Autodesk Inventor part; units mm, degrees
ref_plane "YZ Plane" through (0, 0, 0) normal (1, 0, 0) x (0, 1, 0)
ref_plane "XZ Plane" through (0, 0, 0) normal (0, 1, 0) x (-1, 0, 0)
ref_plane "XY Plane" through (0, 0, 0) normal (0, 0, 1) x (1, 0, 0)
sketch "Sketch4" plane through (0, 0, 0) normal (0, 1, 0) x (-1, 0, 0)
  line L0 (17, 17) -> (-17, 17)
  line L1 (-17, 17) -> (-17, -17)
  line L2 (-17, -17) -> (17, -17)
  line L3 (17, -17) -> (17, 17)
  line L4 (17, 17) -> (-17, -17) construction
  line L5 (-17, 17) -> (17, -17) construction
  point P0 (0, 0)
  dimension "d52" = 34
  dimension "d53" = 34
extrude "Extrusion5" add sketch "Sketch4" along normal blind 2
sketch "Sketch6" plane through (0, 0, 0) normal (0, -1, 0) x (1, 0, 0)
  line L0 (-16.5, -10) -> (-15.5, -10)
  line L1 (-15.5, -10) -> (-15.5, 10)
  line L2 (-15.5, 10) -> (-16.5, 10)
  line L3 (-16.5, 10) -> (-16.5, -10)
  line L4 (-15.5, -10) -> (-16.5, -10)
  line L5 (-16.5, -10) -> (-16.5, 10)
  line L6 (-16.5, 10) -> (-15.5, 10)
  line L7 (-15.5, 10) -> (-15.5, -10)
  line L8 (-10, 16.5) -> (10, 16.5)
  line L9 (10, 16.5) -> (10, 15.5)
  line L10 (10, 15.5) -> (-10, 15.5)
  line L11 (-10, 15.5) -> (-10, 16.5)
  line L12 (10, 16.5) -> (-10, 16.5)
  line L13 (-10, 16.5) -> (-10, 15.5)
  line L14 (-10, 15.5) -> (10, 15.5)
  line L15 (10, 15.5) -> (10, 16.5)
  line L16 (15.5, 10) -> (16.5, 10)
  line L17 (16.5, 10) -> (16.5, -10)
  line L18 (16.5, -10) -> (15.5, -10)
  line L19 (15.5, -10) -> (15.5, 10)
  line L20 (15.5, -10) -> (16.5, -10)
  line L21 (16.5, -10) -> (16.5, 10)
  line L22 (16.5, 10) -> (15.5, 10)
  line L23 (15.5, 10) -> (15.5, -10)
  line L24 (10, -15.5) -> (-10, -15.5)
  line L25 (-10, -15.5) -> (-10, -16.5)
  line L26 (-10, -16.5) -> (10, -16.5)
  line L27 (10, -16.5) -> (10, -15.5)
  line L28 (-10, -15.5) -> (10, -15.5)
  line L29 (10, -15.5) -> (10, -16.5)
  line L30 (10, -16.5) -> (-10, -16.5)
  line L31 (-10, -16.5) -> (-10, -15.5)
  line L32 (-17, 17) -> (-17, -17)
  line L33 (17, 17) -> (-17, 17)
  line L34 (17, -17) -> (17, 17)
  line L35 (-17, -17) -> (17, -17)
  line L36 (17, 17) -> (17, -17)
  line L37 (-17, -17) -> (-17, 17)
  line L38 (-17, 17) -> (17, 17)
  line L39 (17, -17) -> (-17, -17)
  point P0 (0, 0)
  point P1 (-16, 10)
  point P2 (-16, -10)
  point P3 (16, 10)
  point P4 (16, -10)
  point P5 (-10, -16)
  point P6 (-16, -10)
  dimension "d123" = 1
  dimension "d124" = 20
  dimension "d119" = 1
  dimension "d118" = 20
  dimension "d116" = 20
  dimension "d117" = 1
  dimension "d112" = 20
  dimension "d113" = 1
  dimension "d108" = 1
  dimension "d109" = 20
  dimension "d104" = 1
  dimension "d105" = 20
  dimension "d101" = 20
  dimension "d102" = 1
  dimension "d97" = 20
  dimension "d98" = 1
  dimension "d114" = 7
  dimension "d115" = 0.5
  dimension "d111" = 0.5
  dimension "d110" = 7
  dimension "d107" = 7
  dimension "d106" = 0.5
  dimension "d103" = 0.5
  dimension "d95" = 7
  dimension "d99" = 7
  dimension "d100" = 0.5
  dimension "d96" = 0.5
  dimension "d94" = 7
  dimension "d93" = 7
  dimension "d122" = 0.5
  dimension "d120" = 7
  dimension "d121" = 0.5
  dimension "d133" = 0
  dimension "d134" = 0
  dimension "d135" = 0
  dimension "d136" = 0
extrude "Extrusion7" add sketch "Sketch6" along normal blind 1 contours L3 L2 L1 L0 | L8 L9 L10 L11 | L16 L17 L18 L19 | L27 L26 L25 L24
fillet "Fillet9" radius 1 1 edges at (17, 1, -17)
fillet "Fillet10" radius 1 1 edges at (-17, 1, -17)
fillet "Fillet11" radius 1 1 edges at (-17, 1, 17)
fillet "Fillet12" radius 1 1 edges at (17, 1, 17)
fillet "Fillet13" radius 1 8 edges at (-16.7071, 2, -16.7071) (-17, 2, 0) (-16.7071, 2, 16.7071) (0, 2, 17) (16.7071, 2, 16.7071) (17, 2, 0) (16.7071, 2, -16.7071) (0, 2, -17)
properties part number "block_main" material "PC/ABS Plastic"
Can you work these out from the model? Positions are in its coordinate system, mm. A direction names the side the tool comes from. Give positions to 0.01 mm unless a question says otherwise; leave off trailing zeros. Write each loop counter-clockwise with the first axis right and the second up, starting at its lowest first coordinate (ties: lowest second). Pieces come first, ordered by that corner, then holes. Notation, with made-up numbers: (23, -18) -> (43, -18) arc R30 ccw to (43, 7) -> close; hole circle Ø8 at (-9.5, 36.25). An arc over 180 degrees is marked (long way). Answer as a JSON object with one key per item and string values. Group by question number.
Item 1: We'd pull the mould along X, two halves only. Please class faces 6 (the face through (-15.5, -0.5, -0.1)), 7 (the face through (0.1, -0.5, 15.5)), 8 (the face through (16.5, -0.5, 0.1)): +X half, -X half, draft (parallel to the pull), parting line (faces both ways), or undercut.
Item 2: For faces 1 (the face through (-16, -0.5, 10)), 2 (the face through (16.699, 1.715, -0.224)), 3 (the face through (0.1, -0.5, -15.5)), 4 (the face through (-16, -0.5, -10)), 5 (the face through (16, -1, 0)), which set-ups out of +Z, -Z, +X, -X, +Y, -Y let a thin tool reach every point of the face, with its end or its side?
Item 3: Suppose I cut it at C-C (y = 1.6). Please give me the cut outline in (x, z).
Item 4: I'm going to push flat-ended pins straight in: P1, Ø0.5, axis at y = -0.5, z = 16, coming from the +X side; P2, Ø3, axis at x = -8, z = -9.5, coming from the -Y side; P3, Ø0.8, axis at x = -16, y = -0.5, coming from the +Z side. Where does each tip first touch, or does it pass through?
Item 5: Please list where these lines run through material, in increasing order: line 1 (Z direction, x = 9, y = -0.15); line 2 (Y direction, x = 2, z = -11). Write a range as [from, to].
Item 6: Suppose I cut it at D-D (x = 4). Please give me the cut outline in (y, z), plus the area to 3 significant figures.
Item 7: Suppose I cut it at A-A (y = -0.4). Please give me the cut outline in (x, z), plus the area to 3 significant figures.
Item 8: Suppose I cut it at B-B (z = 8). Please give me the cut outline in (x, y), plus the area to 3 significant figures.
Findings:
{
 "1": {"face 6": "undercut", "face 7": "draft", "face 8": "+X half"},
 "2": {"face 1": "+Z, +X, -X, -Y", "face 2": "+Z, -Z, +X, +Y", "face 3": "+X, -X, -Y", "face 4": "-Z, +X, -X, -Y", "face 5": "+Z, -Z, +X, -X, -Y"},
 "3": {"outline": "(-16.8, -16) arc R0.8 ccw to (-16, -16.8) -> (16, -16.8) arc R0.8 ccw to (16.8, -16) -> (16.8, 16) arc R0.8 ccw to (16, 16.8) -> (-16, 16.8) arc R0.8 ccw to (-16.8, 16) -> close"},
 "4": {"P1": "stops at x = 10", "P2": "stops at y = 0", "P3": "stops at z = 10"},
 "5": {"line 1": "z = [-16.5, -15.5], [15.5, 16.5]", "line 2": "y = [0, 2]"},
 "6": {"outline": "(-1, -16.5) -> (0, -16.5) -> (0, -17) -> (1, -17) arc R1 ccw to (2, -16) -> (2, 16) arc R1 ccw to (1, 17) -> (0, 17) -> (0, 16.5) -> (-1, 16.5) -> (-1, 15.5) -> (0, 15.5) -> (0, -15.5) -> (-1, -15.5) -> close", "area": "69.6 mm²"},
 "7": {"outline": "(-16.5, -10) -> (-15.5, -10) -> (-15.5, 10) -> (-16.5, 10) -> close; (-10, -16.5) -> (10, -16.5) -> (10, -15.5) -> (-10, -15.5) -> close; (-10, 15.5) -> (10, 15.5) -> (10, 16.5) -> (-10, 16.5) -> close; (15.5, -10) -> (16.5, -10) -> (16.5, 10) -> (15.5, 10) -> close", "area": "80.0 mm²"},
 "8": {"outline": "(-17, 0) -> (-16.5, 0) -> (-16.5, -1) -> (-15.5, -1) -> (-15.5, 0) -> (15.5, 0) -> (15.5, -1) -> (16.5, -1) -> (16.5, 0) -> (17, 0) -> (17, 1) arc R1 ccw to (16, 2) -> (-16, 2) arc R1 ccw to (-17, 1) -> close", "area": "69.6 mm²"}
}
